Could you check a few things on this drawing? It's one solid part, dimensions in mm from its lowest x, y, z. A direction names the side the tool comes from. Round coordinates to 2 decimals unless told otherwise and drop trailing zeros. Write each loop counter-clockwise with the first axis right and the second up, starting at its lowest first coordinate (ties: lowest second). Pieces come first, ordered by that corner, then holes. Notation, with made-up numbers: (66.5, -5) -> (71.5, -5) arc R25 cw to (71.5, 9) -> close; hole circle Ø6 at (-28, 81.25). An arc over 180 degrees is marked (long way). Return JSON: item names as keys, results as strings.
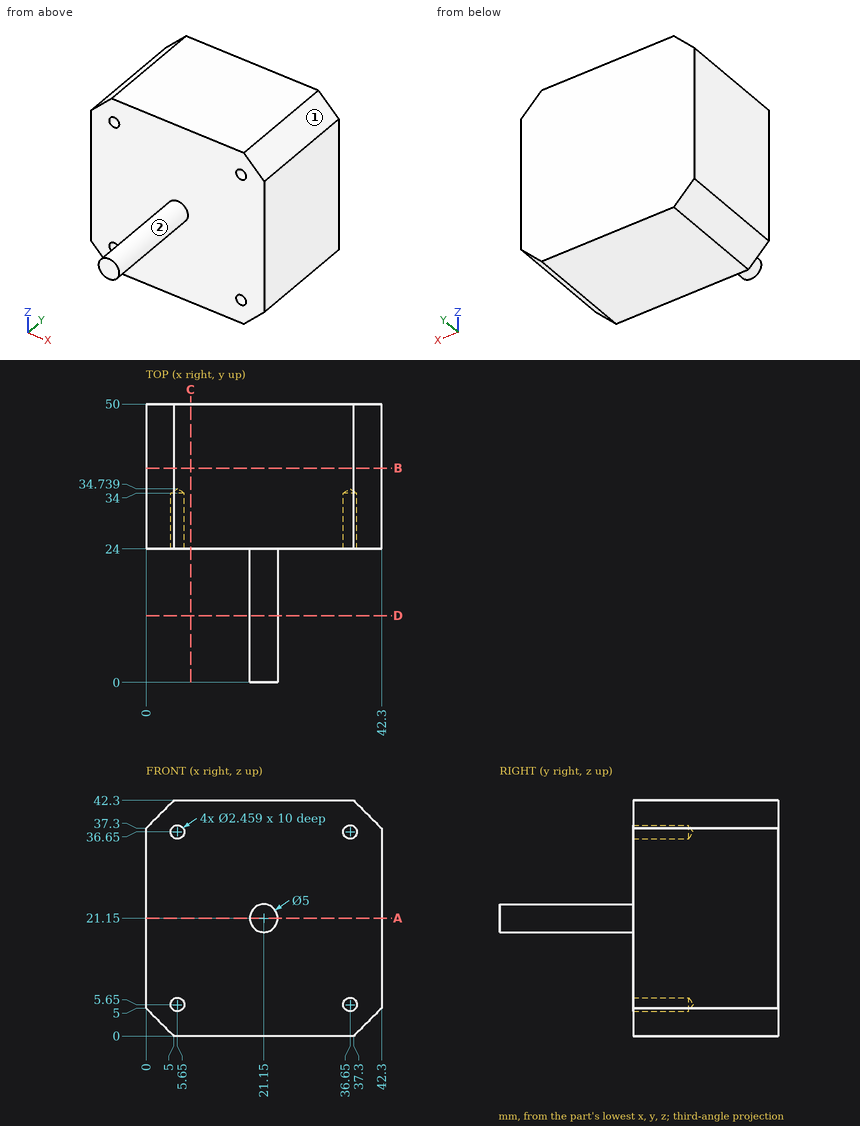
1) Will these pins go through, and if not, where does the flat tip stop? pin 1 Ø2 at (x, z) = (5.65, 5.65) entering from -Y; pin 2 Ø6 at (x, y) = (25, 18) entering from -Z; pin 3 Ø6 at (x, y) = (24, 11.5) entering from -Z.
Return value:
{"pin 1": "y = 34.14", "pin 2": "z = 18.8", "pin 3": "z = 18.65"}
2) For the marked faces 1 and 2, which set-ups out of +Z, -Z, +X, -X, +Y, -Y let a thin tool reach every point of the face, with its end or its side?
Return value:
{"face 1": "+Z, +X, +Y, -Y", "face 2": "-Y"}
3) I want a section at B-B, the plane y = 38.5. Please give me the cut outline in (x, z).
Return value:
{"outline": "(0, 5) -> (5, 0) -> (37.3, 0) -> (42.3, 5) -> (42.3, 37.3) -> (37.3, 42.3) -> (5, 42.3) -> (0, 37.3) -> close"}
4) I want a section at C-C, the plane x = 8. Please give me the cut outline in (y, z).
Return value:
{"outline": "(24, 0) -> (50, 0) -> (50, 42.3) -> (24, 42.3) -> close"}
5) If I drill on probe 1 along X at (y, z) = (27.5, 5.65); probe 2 along Z at (x, y) = (5, 29) (1 decimal), over which ranges is the centre line in solid material (lowest first)? Write a range as [from, to].
Return value:
{"probe 1": "[0, 4.42], [6.88, 35.42], [37.88, 42.3]", "probe 2": "[0, 4.6], [6.7, 35.6], [37.7, 42.3]"}
6) I want a section at D-D, the plane y = 12. Please give me the cut outline in (x, z), and give its area (3 significant figures).
Return value:
{"outline": "circle Ø5 at (21.15, 21.15)", "area": "19.6 mm²"}
7) I want a section at A-A, the plane z = 21.15. Please give me the cut outline in (x, y).
Return value:
{"outline": "(0, 24) -> (18.65, 24) -> (18.65, 0) -> (23.65, 0) -> (23.65, 24) -> (42.3, 24) -> (42.3, 50) -> (0, 50) -> close"}
